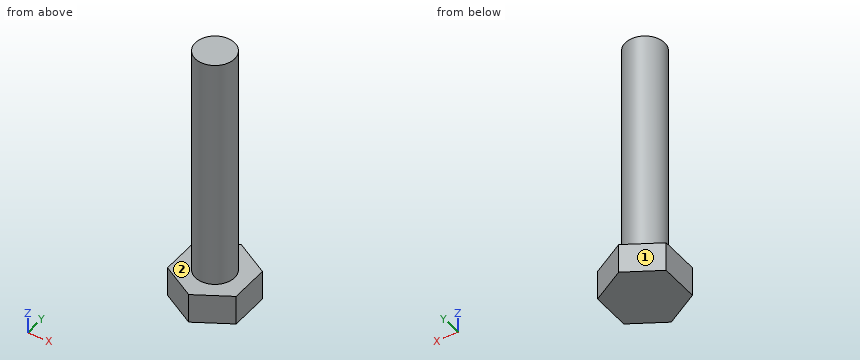
from build123d import *

# Parameters (mm, degrees)
SKETCH_R     = 3.175
PAD_DEPTH    = 38.1
PAD001_DEPTH = 4.8


with BuildPart() as part:
    # Sketch → Pad (new body)
    with BuildSketch(Plane.XY):
        Circle(SKETCH_R)
    extrude(amount=PAD_DEPTH)

    # Sketch001 → Pad001 (join)
    with BuildSketch(Plane.XY):
        Polygon((0, 6.425908), (-5.565, 3.212954), (-5.565, -3.212954), (0, -6.425908), (5.565, -3.212954), (5.565, 3.212954), align=None)
    extrude(amount=-PAD001_DEPTH)


solid = part.part
Design review of the part built by this model. Coordinates are the model's own, in mm. Face numbers are marked on the shaded views. A direction names the side the tool comes from. Round coordinates to 2 decimals unless told otherwise and drop trailing zeros. Write each loop counter-clockwise with the first axis right and the second up, starting at its lowest first coordinate (ties: lowest second). Pieces come first, ordered by that corner, then holes.
Item 1: Consider section D-D on y = 2.75. Give the boundary of the cut face in (x, z) (3 decimals), and give its area (3 significant figures).
Item 2: Consider section C-C on x = 4. Give the boundary of the cut face in (y, z).
Item 3: For the marked faces 1 and 2, list the 3-axis set-ups (+Z, -Z, +X, -X, +Y, -Y) from which the entire face can be reached by the end or side of a thin tool; tool diameter is ignored.
Item 4: Consider section B-B on z = 31.5. Give the boundary of the cut face in (x, y) (3 decimals), and give its area (3 significant figures).
Item 5: Wall thickness on L1, parallel to Z at x = 3, y = 3.25; L2, parallel to X at y = -0.25, z = 1.5; L3, parallel to X at y = 1, z = 8: over which ranges is each line inside the solid? List them lowest first.
Item 6: Consider section A-A on y = 0. Give the boundary of the cut face in (x, z) (3 decimals).
Item 7: For pin 1 Ø6 at (x, z) = (-2, 33.5) entering from +Y (3 decimals); pin 2 Ø5 at (y, z) = (2.5, 33) entering from -X (3 decimals), all flat-tipped, find the tip position at first contact; note any pin that passes through.
Check values:
1. outline: (-5.565, -4.8) - (5.565, -4.8) - (5.565, 0) - (1.587, 0) - (1.587, 38.1) - (-1.587, 38.1) - (-1.587, 0) - (-5.565, 0) - close
1. area: 174 mm2
2. outline: (-4.12, -4.8) - (4.12, -4.8) - (4.12, 0) - (-4.12, 0) - close
3. face 1: +Z, -Z, -X, +Y
3. face 2: +Z
4. outline: circle Ø6.35 at (0, 0)
4. area: 31.7 mm2
5. L1: z = -4.8 to 0
5. L2: x = -3.17 to 3.17
5. L3: x = -3.01 to 3.01
6. outline: (-5.565, -4.8) - (5.565, -4.8) - (5.565, 0) - (3.175, 0) - (3.175, 38.1) - (-3.175, 38.1) - (-3.175, 0) - (-5.565, 0) - close
7. pin 1: stops at y = 3.175
7. pin 2: stops at x = -3.175
